For this review, take the finished solid that the model builds, in its own axes (mm). A direction names the side the tool comes from. Give positions to 0.01 mm unless a question says otherwise; leave off trailing zeros. Loops run counter-clockwise (first coordinate to the right, second up) from the corner with the lowest first, then second, coordinate; pieces in that order, holes last.
```python
from build123d import *

# Parameters (mm, degrees)
SKETCH1_R           = 0.95
SKETCH1_R_2         = 0.381
BOSS_EXTRUDE1_DEPTH = 3
BOSS_EXTRUDE2_START = 4
SKETCH2_R           = 4.43
SKETCH2_R_2         = 2.43
BOSS_EXTRUDE2_DEPTH = 4


with BuildPart() as part:
    # Sketch1 → Boss-Extrude1 (new body)
    with BuildSketch(Plane.XY):
        with BuildLine():
            Line((0.94968125, 4.327008843), (16.214375, 0.976751432))
            ThreePointArc((16.214375, 0.976751432), (17, 0), (16.214375, -0.976751432))
            Line((16.214375, -0.976751432), (0.94968125, -4.327008843))
            ThreePointArc((0.94968125, -4.327008843), (-4.43, 0), (0.94968125, 4.327008843))
        make_face()
        Circle(SKETCH1_R, mode=Mode.SUBTRACT)
        with Locations((16, 0)):
            Circle(SKETCH1_R_2, mode=Mode.SUBTRACT)
    extrude(amount=BOSS_EXTRUDE1_DEPTH)

    # Sketch2 → Boss-Extrude2 (add)
    with BuildSketch(Plane(origin=(0, 0, 0), x_dir=(-1, 0, 0), z_dir=(0, 0, -1)).offset(BOSS_EXTRUDE2_START)):
        Circle(SKETCH2_R)
        Circle(SKETCH2_R_2, mode=Mode.SUBTRACT)
    extrude(amount=-BOSS_EXTRUDE2_DEPTH)


solid = part.part
```
Item 1: The part is to be moulded in two halves that separate along Y. For faces 1 (the flat face through (8.69, -2.63, 1.48)), 2 (the flat face through (9, 0, 0)), 3 (the flat face through (8.475, 2.675, 1.479)), 4 (the cylindrical face through (1.928, -1.479, -2.028)), say which applies: released by +Y, released by -Y, zero draft, split by the parting line, or undercut.
Answer:
face 1: released by -Y
face 2: zero draft
face 3: released by +Y
face 4: undercut
Item 2: Take a section at A-A on x = 16. Give the boundary of the cut face in (y, z), and give its area (3 significant figures).
Answer:
outline: (-1.02, 0) - (-0.38, 0) - (-0.38, 3) - (-1.02, 3) - close; (0.38, 0) - (1.02, 0) - (1.02, 3) - (0.38, 3) - close
area: 3.86 mm2
Item 3: Clearance check with flat-ended pins moving along their axes: pin 1 Ø1.7 at (x, y) = (0, 0) entering from +Z; pin 2 Ø2.5 at (x, y) = (9, -1) entering from -Z; pin 3 Ø1.5 at (y, z) = (1.5, 0) entering from +X. State where each tip first meets the part, or that it passes through.
Answer:
pin 1: passes through
pin 2: stops at z = 0
pin 3: stops at x = 16.66
Item 4: Take a section at C-C on y = 3.25. Give the boundary of the cut face in (x, z), and give its area (3 significant figures).
Answer:
outline: (-3.01, -4) - (3.01, -4) - (3.01, 0) - (5.86, 0) - (5.86, 3) - (-3.01, 3) - close
area: 50.7 mm2
Item 5: For L1, parallel to Y at x = 0, z = -2.25; L2, parallel to X at y = -1.5, z = -2.25; L3, parallel to Z at x = 11.25, y = -1.5, list the stretches that pass through material, from the lowest coordinate up.
Answer:
L1: y = -4.43 to -2.43, 2.43 to 4.43
L2: x = -4.17 to -1.91, 1.91 to 4.17
L3: z = 0 to 3
Item 6: Tool access review of faces 5 (the flat face through (-2, -2, -4)), 6 (the flat face through (-1, -1, 0)): name each direction out of +Z, -Z, +X, -X, +Y, -Y from which nothing blocks a thin tool from reaching the whole face with its end or side.
Answer:
face 5: -Z, +X, -X, +Y, -Y
face 6: -Z
Item 7: Take a section at B-B on z = 2.5. Give the boundary of the cut face in (x, y).
Answer:
outline: (0.95, -4.33) - (16.21, -0.98) arc R1 ccw to (16.21, 0.98) - (0.95, 4.33) arc R4.43 ccw (long way) to start; hole circle Ø1.9 at (0, 0); hole circle Ø0.76 at (16, 0)
